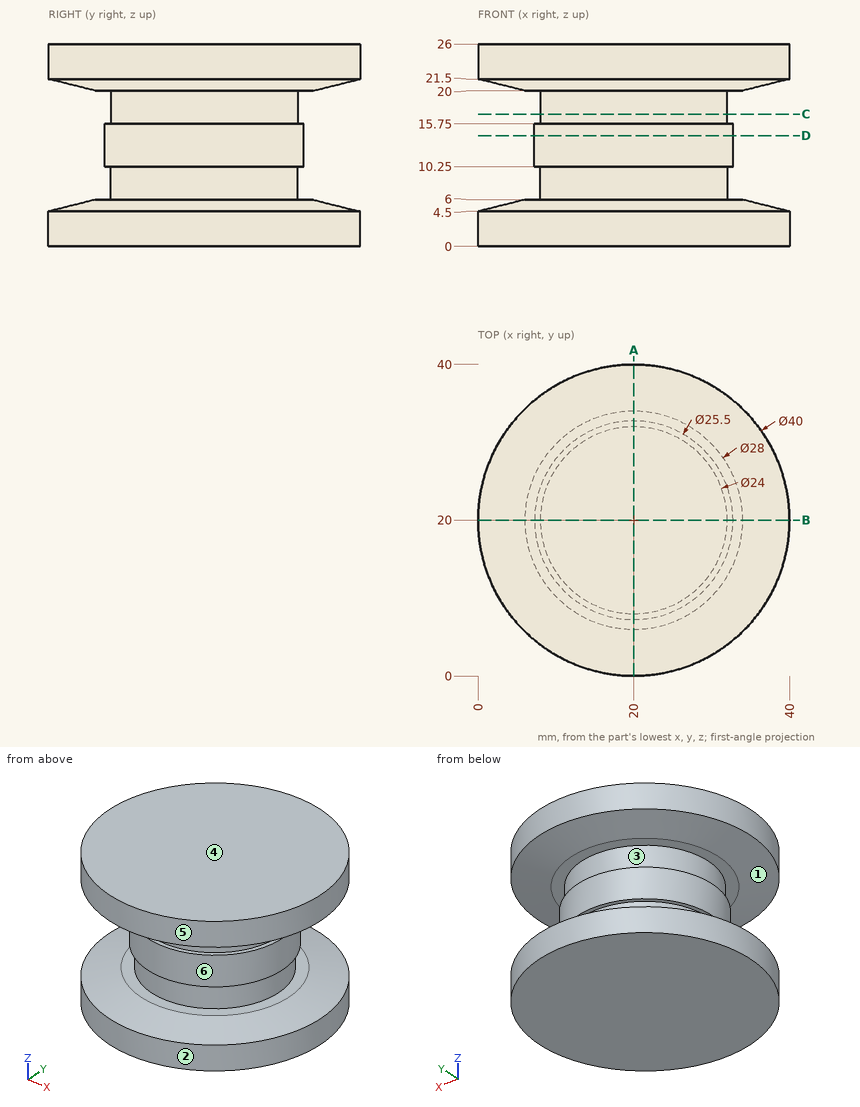
Answer from the drawing. Dimensions are ordinates in mm from the lowest x, y and z of the part. A direction names the side the tool comes from. Coordinates: 2 decimals unless noted, no trailing zeros. Order: outer loops, then holes, each group sorted by start corner. A loop starts at its lowest first (then second) coordinate and runs counter-clockwise, first axis right, second up. Notation, with made-up numbers: (13, 6) - (59, 6) arc R6 ccw to (59, 11) - close; hole circle Ø6 at (35.5, 4). An arc over 180 degrees is marked (long way). Put each result on its own line as item: value. Start each with the question number.
1) Find section D-D (z = 14.25). Give the vertices of the cut face in (x, y), plus the area to 3 significant figures.
2) For the marked faces 5 and 6, determine the directions among +Z, -Z, +X, -X, +Y, -Y from which every point of the face is accessible in a straight line to the end or side of a thin tool.
3) Find section A-A (x = 20). Give the vertices of the cut face in (y, z).
4) For a pull along Z with two mould halves and no side action, classify the marked faces 1, 2, 3 and 4 as released by +Z, released by -Z, zero draft, split by the parting line, or undercut.
5) Find section C-C (z = 17). Give the vertices of the cut face in (x, y), plus the area to 3 significant figures.
6) Find the intervals of material crossed by line 1 (Z direction, x = 6.5, y = 10.5); line 2 (Y direction, x = 28, z = 22); line 3 (X direction, y = 27, z = 19.5), in increasing order. Write a range as from..to.
7) Flat-ended cylindrical pins translate along their axes: pin 1 (2 mm diameter, centred on y = 16, z = 11, fed in from +X); pin 2 (2 mm diameter, centred on x = 10, z = 14, fed in from +Y); pin 3 (8 mm diameter, centred on x = 13, z = 21.5, fed in from +Y). Find the tip coordinate at first contact, or state that the pin passes through.
Results list:
1. outline: circle Ø25.5 at (20, 20)
1. area: 511 mm^2
2. face 5: +Z, -Z
2. face 6: none
3. outline: (0, 0) - (40, 0) - (40, 4.5) - (34, 6) - (32, 6) - (32, 10.25) - (32.75, 10.25) - (32.75, 15.75) - (32, 15.75) - (32, 20) - (34, 20) - (40, 21.5) - (40, 26) - (0, 26) - (0, 21.5) - (6, 20) - (8, 20) - (8, 15.75) - (7.25, 15.75) - (7.25, 10.25) - (8, 10.25) - (8, 6) - (6, 6) - (0, 4.5) - close
4. face 1: undercut
4. face 2: zero draft
4. face 3: undercut
4. face 4: released by +Z
5. outline: circle Ø24 at (20, 20)
5. area: 452 mm^2
6. line 1: z = 0..5.37, 20.63..26
6. line 2: y = 1.67..38.33
6. line 3: x = 10.25..29.75
7. pin 1: stops at x = 32.39
7. pin 2: stops at y = 29.03
7. pin 3: stops at y = 39.77
